Autodesk Inventor part; units mm, degrees
ref_plane "YZ Plane" through (0, 0, 0) normal (1, 0, 0) x (0, 1, 0)
ref_plane "XZ Plane" through (0, 0, 0) normal (0, 1, 0) x (-1, 0, 0)
ref_plane "XY Plane" through (0, 0, 0) normal (0, 0, 1) x (1, 0, 0)
sketch "Sketch1" plane through (0, 0, 0) normal (0, 1, 0) x (-1, 0, 0)
  circle A0 centre (0, 0) radius 10.375
  arc A1 (15.885, 1.9145) -> (15.9655, -1.0494) centre (15.6971, 0.4263) ccw
  arc A2 (6.2845, 14.7141) -> (8.8916, 13.3018) centre (7.4793, 13.8073) ccw
  arc A3 (-9.6005, 12.7996) -> (-7.0739, 14.3513) centre (-8.2178, 13.3809) ccw
  arc A4 (-15.885, -1.9145) -> (-15.9655, 1.0494) centre (-15.6971, -0.4263) ccw
  arc A5 (-6.2845, -14.7141) -> (-8.8916, -13.3018) centre (-7.4793, -13.8073) ccw
  arc A6 (9.6005, -12.7996) -> (7.0739, -14.3513) centre (8.2178, -13.3809) ccw
  arc A7 (9.6005, -12.7996) -> (15.9655, -1.0494) centre (0, 0) ccw
  arc A8 (-6.2845, -14.7141) -> (7.0739, -14.3513) centre (0, 0) ccw
  arc A9 (-15.885, -1.9145) -> (-8.8916, -13.3018) centre (0, 0) ccw
  arc A10 (-9.6005, 12.7996) -> (-15.9655, 1.0494) centre (0, 0) ccw
  arc A11 (15.885, 1.9145) -> (8.8916, 13.3018) centre (0, 0) ccw
  arc A12 (6.2845, 14.7141) -> (-7.0739, 14.3513) centre (0, 0) ccw
  dimension "d0" = 20.75
  dimension "d4" = 3
  dimension "d7" = 360
  dimension "d10" = 16
extrude "Extrusion1" add sketch "Sketch1" along normal blind 8
fillet "Fillet1" radius 2 12 edges at (9.6005, 4, 12.7996) (15.9655, 4, 1.0494) (15.885, 4, -1.9145) (8.8916, 4, -13.3018) (6.2845, 4, -14.7141) (-7.0739, 4, -14.3513) (-9.6005, 4, -12.7996) (-15.9655, 4, -1.0494) (-15.885, 4, 1.9145) (-8.8916, 4, 13.3018) (-6.2845, 4, 14.7141) (7.0739, 4, 14.3513)
sketch "Sketch2" plane through (0, 0, 0) normal (0, -1, 0) x (1, 0, 0)
  circle A0 centre (0, 0) radius 10.375
  circle A1 centre (0, 0) radius 12.5
  dimension "d11" = 25
extrude "Extrusion2" cut sketch "Sketch2" against normal blind 3
properties part number "springSpacerV1"
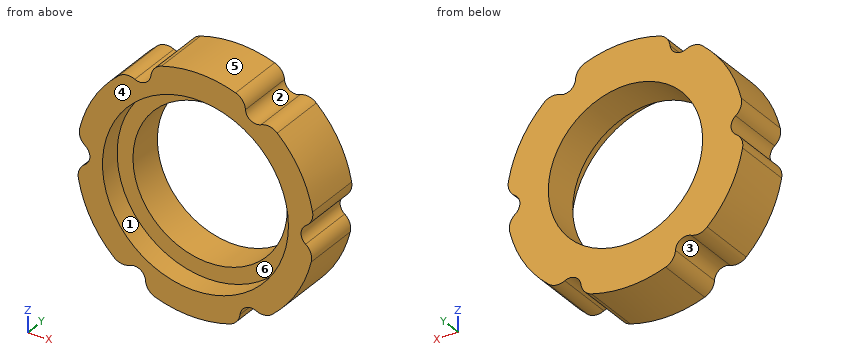
Model file for the job. Use its own axes, mm. Face numbers are marked on the shaded views. A direction names the side the tool comes from. Round coordinates to 2 decimals unless told otherwise and drop trailing zeros. Order: outer loops, then holes, each group sorted by start corner. A loop starts at its lowest first (then second) coordinate and runs counter-clockwise, first axis right, second up. Notation, with made-up numbers: M -2.75,-4.5 L 54.25,-4.5 A7 cw 54.25,7.5 Z; hole C 66.5,27 d4. An arc over 180 degrees is marked long. Write each question's results on one line, items separated by ' | '. Start each with the question number.
(1) Which spindle directions (+Z, -Z, +X, -X, +Y, -Y) get a long thin tool onto all of the face, cutting with end or side? Do the marked faces 5 and 6. Say none if no direction does.
(2) Two-plate mould, pull along Z, no slides. Class the marked faces 1, 2, 3 and 4: pulls with the +Z half, pulls with the -Z half, needs draft (parallel to the pull), parting line crosses it, or undercut.
(3) Saw through at A-A, the plane x = 0. Give the cut face in (y, z) (3 decimals), then the cut area to 4 significant figures.
(4) Saw through at B-B, the plane z = 6. Give the cut face in (x, y).
(5) Drop flat-ended pins along their axis: pin 1 (1.5 mm diameter, centred on x = -6.5, z = 6.5, fed in from +Y); pin 2 (2 mm diameter, centred on x = 12.5, y = 1, fed in from -Z); pin 3 (4 mm diameter, centred on y = 2, z = 7.5, fed in from +X); pin 4 (1.5 mm diameter, centred on x = 12.5, y = 6.5, fed in from +Z). Give the stop position or say it passes through.
(6) Probe probe 1 along Z at (x, y) = (0, 0.7); probe 2 along Z at (x, y) = (0, 7) (3 decimals); probe 3 along X at (y, z) = (6.25, 4). List the from-to ranges inside material, lowest first. Write a range as from..to.
Established:
1) face 5: +Z, +Y, -Y | face 6: -Y
2) face 1: undercut | face 2: pulls with the +Z half | face 3: pulls with the -Z half | face 4: needs draft
3) outline: M 0,-16 L 8,-16 L 8,-10.375 L 3,-10.375 L 3,-12.5 L 0,-12.5 Z; M 0,12.5 L 3,12.5 L 3,10.375 L 8,10.375 L 8,16 L 0,16 Z | area: 77.25 mm^2
4) outline: M -14.83,0 L -10.97,0 L -10.97,3 L -8.46,3 L -8.46,8 L -14.83,8 Z; M 8.46,3 L 10.97,3 L 10.97,0 L 14.83,0 L 14.83,8 L 8.46,8 Z
5) pin 1: passes through | pin 2: stops at z = -11.12 | pin 3: stops at x = 15.02 | pin 4: stops at z = 10.86
6) probe 1: z = -16..-12.5, 12.5..16 | probe 2: z = -16..-10.375, 10.375..16 | probe 3: x = -15.49..-9.57, 9.57..15.49
